Autodesk Inventor part; units mm, degrees
ref_plane "Work Plane2" through (0, 494.5349, 0) normal (0, 1, 0) x (-1, 0, 0)
ref_plane "YZ Plane" through (0, 0, 0) normal (1, 0, 0) x (0, 1, 0)
ref_plane "XY Plane" through (0, 0, 0) normal (0, 0, 1) x (1, 0, 0)
ref_plane "Work Plane2" through (0, 494.5349, 0) normal (0, 1, 0) x (-1, 0, 0)
sketch "Sketch1" plane through (0, 494.5349, 0) normal (0, 1, 0) x (-1, 0, 0)
  circle A0 centre (-3068.8365, 412.4332) radius 3.2
  line L0 (614.5573, 0) -> (-3687.3438, 0)
  line L1 (0, -83.2766) -> (0, 499.6599)
  circle A1 centre (-3068.8365, 412.4332) radius 3.95
  point P0 (0, 0)
  dimension "d2" = 6.4
  dimension "d3" = 412.4332
  dimension "d4" = 3068.8364
  dimension "d7" = 7.9
extrude "Extrusion1" add sketch "Sketch1" against normal blind 21.4 contours A0 | A1
sketch "Sketch2" plane through (3068.8365, 473.1349, 412.4332) normal (0, -1, 0) x (1, 0, 0)
  circle A0 centre (0, 0) radius 3.95
  circle A1 centre (0, 0) radius 5.715
  dimension "d8" = 11.43
extrude "Extrusion2" add sketch "Sketch2" along normal blind 1.52 contours A0 | A1
fillet "Fillet1" radius 0.25 1 edges at (3072.7865, 473.1349, 412.4332)
chamfer "Chamfer2" distance 1.27 distance2 0.7554 1 edges at (3072.7865, 494.5349, 412.4332) measured on face at (3068.0463, 480.4349, 416.3034)
properties part number "313-04" material "Steel, High Strength Low Alloy"
Check sheet for the modelled part. Datum: model origin and axes. Units: mm. A direction names the side the tool comes from. Give positions to 0.01 mm unless a question says otherwise; leave off trailing zeros. Write each loop counter-clockwise with the first axis right and the second up, starting at its lowest first coordinate (ties: lowest second). Pieces come first, ordered by that corner, then holes. Notation, with made-up numbers: (-17.5, 62) - (12.5, 62) arc R26 cw to (12.5, 85) - close; hole circle Ø6 at (23.25, 27.5). An arc over 180 degrees is marked (long way). Answer as a JSON object with one key per item and string values. Group by question number.
1) Thickness scan on probe 1 along Y at (x, z) = (3069, 417); probe 2 along Z at (x, y) = (3069, 484); probe 3 along Z at (x, y) = (3071.75, 488). Record the ranges inside material, lowest first. Write a range as from..to.
2) Sectioned sample at A-A (y = 480.25). Record the cut outline in (x, z).
3) Access from +Z, -Z, +X, -X, +Y, -Y to the whole of each face (thin tool, end or side, straight path). Record for faces 1 (the face through (3069, 471.615, 413)), 2 (the face through (3072.783, 483.464, 412.607)).
4) Depth check by flat-ended pin: P1, Ø4, axis at x = 3067, y = 478.5, coming from the -Z side; P2, Ø4, axis at x = 3065.5, z = 416.5, coming from the +Y side; P3, Ø6, axis at x = 3065, y = 481.5, coming from the +Z side. Enter the tip coordinate at first touch or a pass-through.
Geometry results:
{
 "1": {"probe 1": "y = 471.61..473.13", "probe 2": "z = 408.49..416.38", "probe 3": "z = 409.77..415.1"},
 "2": {"outline": "circle Ø7.9 at (3068.84, 412.43)"},
 "3": {"face 1": "+Z, -Z, +X, -X, -Y", "face 2": "+Y"},
 "4": {"P1": "stops at z = 408.48", "P2": "stops at y = 494.42", "P3": "stops at z = 416.29"}
}
